Work out the finished part from the listing and answer in its coordinate system (mm). A direction names the side the tool comes from. Coordinates: 2 decimals unless noted, no trailing zeros. Order: outer loops, then holes, each group sorted by start corner. A loop starts at its lowest first (then second) coordinate and runs counter-clockwise, first axis right, second up. Notation, with made-up numbers: M 88.25,48.25 L 144.25,48.25 A25 cw 144.25,73.25 Z; hole C 29,85.5 d4. An arc over 180 degrees is marked long. Use a Markdown table: item, result.
Solid Edge part; units mm, degrees
sketch "Sketch1" plane through (0, 0, 0) normal (0, -1, 0) x (1, 0, 0)
  line L0 (30, 0) -> (65, 52)
  line L1 (65, 52) -> (90, 52)
  line L2 (90, 52) -> (90, 60)
  line L3 (90, 60) -> (56.9204, 60)
  line L4 (56.9204, 60) -> (0, 60)
  line L5 (0, 60) -> (0, 52)
  line L6 (0, 52) -> (23, 52)
  line L7 (23, 52) -> (23, 8)
  line L8 (23, 8) -> (0, 8)
  line L9 (0, 8) -> (0, 0)
  line L10 (0, 0) -> (30, 0)
  dimension "D1" = 23
extrude "Protrusion1" add sketch "Sketch1" against normal blind 50
mirror "Mirror1" about plane through (0, 25, 4) normal (-1, 0, 0) of "Protrusion1"
sketch "Sketch2" plane through (0, 0, 26) normal (0, -1, 0) x (1, 0, 0)
  line L0 (30, -16.6796) -> (58.7267, 26)
  line L1 (58.7267, 26) -> (30, 26)
  line L2 (30, 26) -> (30, -16.6796)
extrude "Cutout1" cut sketch "Sketch2" against normal through all
sketch "Sketch3" plane through (0, 25, 0) normal (0, 0, -1) x (1, 0, 0)
  circle A0 centre (-16, 21) radius 1.65
  circle A1 centre (16, 21) radius 1.65
  circle A2 centre (16, -21) radius 1.65
  circle A3 centre (-16, -21) radius 1.65
extrude "Cutout2" cut sketch "Sketch3" against normal up to next
sketch "Sketch4" plane through (0, 25, 8) normal (0, 0, 1) x (1, 0, 0)
  circle A0 centre (-16, -21) radius 3.75
  circle A1 centre (16, -21) radius 3.75
  circle A2 centre (-16, 21) radius 3.75
  circle A3 centre (16, 21) radius 3.75
extrude "Extrusionsausschnitt_4" cut sketch "Sketch4" against normal blind 5
sketch "Sketch5" plane through (0, 25, 60) normal (0, 0, 1) x (-1, 0, 0)
  circle A0 centre (-62.5, 20) radius 1.4
  circle A1 centre (-62.5, -20) radius 1.4
  circle A2 centre (62.5, -20) radius 1.4
  circle A3 centre (62.5, 20) radius 1.4
  dimension "D1" = 62.5
  dimension "D2" = 62.5
extrude "Cutout3" cut sketch "Sketch5" against normal through all
mirror "Mirror2" about plane through (0, 0, 0) normal (1, 0, 0) of "Cutout1"
properties material "Nylon, allgemein"
(1) A cutting plane is placed at D-D (x = -55.5). Determine the outline of the cut face in (y, z), then the cut area to 3 significant figures.
Conclusion:
| item | result |
|---|---|
| outline | M 0,37.89 L 50,37.89 L 50,47.21 L 0,47.21 Z; M 0,52 L 50,52 L 50,60 L 0,60 Z |
| area | 866 mm2 |
(2) A cutting plane is placed at A-A (x = 16). Determine the outline of the cut face in (y, z), then the cut area to 3 significant figures.
Conclusion:
| item | result |
|---|---|
| outline | M 0,0 L 2.35,0 L 2.35,3 L 0.25,3 L 0.25,8 L 0,8 Z; M 0,52 L 50,52 L 50,60 L 0,60 Z; M 5.65,0 L 44.35,0 L 44.35,3 L 42.25,3 L 42.25,8 L 7.75,8 L 7.75,3 L 5.65,3 Z; M 47.65,0 L 50,0 L 50,8 L 49.75,8 L 49.75,3 L 47.65,3 Z |
| area | 705 mm2 |
(3) A cutting plane is placed at C-C (z = 40.5). Determine the outline of the cut face in (x, y), then the cut area to 3 significant figures.
Conclusion:
| item | result |
|---|---|
| outline | M -57.26,0 L -50.99,0 L -50.99,50 L -57.26,50 Z; M -30,0 L -23,0 L -23,50 L -30,50 Z; M 23,0 L 30,0 L 30,50 L 23,50 Z; M 50.99,0 L 57.26,0 L 57.26,50 L 50.99,50 Z |
| area | 1,330 mm2 |
(4) Determine the mould class of faces 4 (the flat face through (90, 25, 56)), 5 (the flat face through (-78, 25, 52)), 6 (the cylindrical face through (15.19, 42.34, 5.54)) for opening direction X: pulls with the +X half, pulls with the -X half, needs draft (parallel to the pull), parting line crosses it, or undercut.
Conclusion:
| item | result |
|---|---|
| face 4 | pulls with the +X half |
| face 5 | needs draft |
| face 6 | undercut |
(5) A cutting plane is placed at B-B (y = 39.5). Determine the outline of the cut face in (x, z).
Conclusion:
| item | result |
|---|---|
| outline | M -90,52 L -65,52 L -30,0 L 30,0 L 65,52 L 90,52 L 90,60 L -90,60 Z; hole M -58.73,52 L -30,9.32 L -30,52 Z; hole M -23,8 L 23,8 L 23,52 L -23,52 Z; hole M 30,9.32 L 58.73,52 L 30,52 Z |
(6) Straight lines are drawn through the part: L1, parallel to Y at x = 16, z = 1.5; L2, parallel to Y at x = -16, z = 5.8; L3, parallel to Z at x = 19, y = 25. For each, find the intervals that lie inside material, in ascending order.
Conclusion:
| item | result |
|---|---|
| L1 | 0 to 2.35, 5.65 to 44.35, 47.65 to 50 |
| L2 | 0 to 0.25, 7.75 to 42.25, 49.75 to 50 |
| L3 | 0 to 8, 52 to 60 |
(7) Given P1, Ø12, axis at y = 8.5, z = 35, coming from the +X side; P2, Ø8, axis at x = -36, y = 23.5, coming from the -Z side; P3, Ø1, axis at y = 12.5, z = 45, coming from the -X side (3 decimals), each flat-ended and moving along its own axis, determine where each tip first touches the part or whether it passes through.
Conclusion:
| item | result |
|---|---|
| P1 | x = 57.6 |
| P2 | z = 2.97 |
| P3 | x = -60.625 |
(8) Which of the six approach directions +Z, -Z, +X, -X, +Y, -Y give full straight-line access (tool end or side, diameter ignored) to faces 1 (the cylindrical face through (-15.11, 44.61, 1.48)), 2 (the flat face through (77, 25, 52)), 3 (the flat face through (23, 25, 30))?
Conclusion:
| item | result |
|---|---|
| face 1 | -Z |
| face 2 | -Z, +X, +Y, -Y |
| face 3 | +Y, -Y |
